CAD build for the part. Positions are in the model's coordinates, mm. Coordinates: 2 decimals unless noted, no trailing zeros. Loops run counter-clockwise (first coordinate to the right, second up) from the corner with the lowest first, then second, coordinate; pieces in that order, holes last. Notation, with made-up numbers: (79.5, 39.25) - (126.5, 39.25) arc R30 cw to (126.5, 66.25) - close; hole circle Ø11 at (46, -31.5). An arc over 180 degrees is marked (long way). Put each result on its own line as item: value.
```python
from build123d import *

# Parameters (mm, degrees)
F0_R     = 38.1
F1_DEPTH = 10.16


with BuildPart() as f1:
    # F0 (on Front) → F1 (new body, symmetric)
    with BuildSketch(Plane.XZ):
        with BuildLine():
            ThreePointArc((93.28624, -121.037828), (68.286859, 0), (93.28624, 121.037828))
            ThreePointArc((93.28624, 121.037828), (0, 262.89), (-93.28624, 121.037828))
            ThreePointArc((-93.28624, 121.037828), (-68.286859, 0), (-93.28624, -121.037828))
            ThreePointArc((-93.28624, -121.037828), (0, -262.89), (93.28624, -121.037828))
        make_face()
        with Locations((0, -161.29)):
            Circle(F0_R, mode=Mode.SUBTRACT)
        with Locations((0, 161.29)):
            Circle(F0_R, mode=Mode.SUBTRACT)
    extrude(amount=F1_DEPTH, both=True)


solid = f1.part
```
Q1. Wall check: L1, parallel to Z at x = 0, y = -4.5; L2, parallel to Z at x = -3, y = -2; L3, parallel to X at y = -6.5, z = -173.5. Give the ranges that are in metal, low to high. Write a range as from..to.
Determined:
L1: -262.89..-199.39, -123.19..123.19, 199.39..262.89
L2: -262.85..-199.27, -123.31..123.31, 199.27..262.85
L3: -100.86..-36.09, 36.09..100.86
Q2. Slice it at C-C, the plane y = 3. Give the cut face in (x, z).
Determined:
outline: (-93.29, -121.04) arc R101.6 ccw (long way) to (93.29, -121.04) arc R305.51 cw to (93.29, 121.04) arc R101.6 ccw (long way) to (-93.29, 121.04) arc R305.51 cw to start; hole circle Ø76.2 at (0, -161.29); hole circle Ø76.2 at (0, 161.29)
Q3. Pin check, flat tips, straight feed: pin 1 Ø4 at (x, y) = (-21, 1) entering from -Z; pin 2 Ø4 at (x, y) = (1.5, 5.5) entering from +Z; pin 3 Ø5 at (y, z) = (7.5, -164) entering from -X. Stop position of each tip, or through.
Determined:
pin 1: z = -261.1
pin 2: z = 262.89
pin 3: x = -101.6
Q4. Slice it at B-B, the plane x = 0. Give the cut face in (y, z), then the cut area to 3 significant figures.
Determined:
outline: (-10.16, -262.89) - (10.16, -262.89) - (10.16, -199.39) - (-10.16, -199.39) - close; (-10.16, -123.19) - (10.16, -123.19) - (10.16, 123.19) - (-10.16, 123.19) - close; (-10.16, 199.39) - (10.16, 199.39) - (10.16, 262.89) - (-10.16, 262.89) - close
area: 7,590 mm2
Q5. Mould opens along X. For faces 1 (the cylindrical face through (-68.29, -0.14, 1.74)), 2 (the flat face through (-1, -10.16, 4)), 3 (the cylindrical face through (-4.96, 0.142, 199.066)), 4 (the cylindrical face through (-4.96, 0.142, -123.514)) say: +X half, -X half, draft (parallel to the pull), parting line (faces both ways), or undercut.
Determined:
face 1: -X half
face 2: draft
face 3: undercut
face 4: undercut
Q6. Slice it at D-D, the plane z = -172. Give the cut face in (x, y), then the cut area to 3 significant figures.
Determined:
outline: (-101.03, -10.16) - (-36.56, -10.16) - (-36.56, 10.16) - (-101.03, 10.16) - close; (36.56, -10.16) - (101.03, -10.16) - (101.03, 10.16) - (36.56, 10.16) - close
area: 2,620 mm2
Q7. Slice it at A-A, the plane z = 161.29. Give the cut face in (x, y).
Determined:
outline: (-101.6, -10.16) - (-38.1, -10.16) - (-38.1, 10.16) - (-101.6, 10.16) - close; (38.1, -10.16) - (101.6, -10.16) - (101.6, 10.16) - (38.1, 10.16) - close
